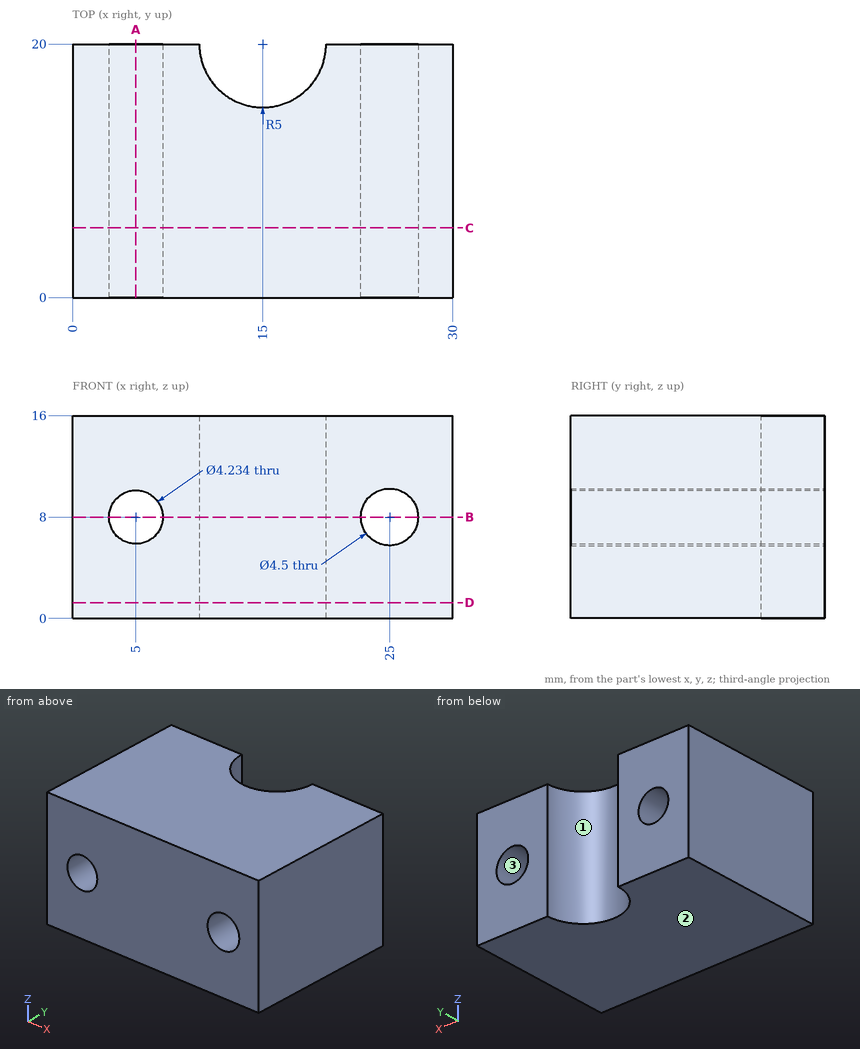
Drawing for the job (mm, zero at the part's lowest x, y, z). Give positions to 0.01 mm unless a question says otherwise; leave off trailing zeros. Order: outer loops, then holes, each group sorted by start corner. A loop starts at its lowest first (then second) coordinate and runs counter-clockwise, first axis right, second up. Notation, with made-up numbers: (88.25, -15) -> (94.25, -15) arc R7 ccw to (94.25, -6) -> close; hole circle Ø11 at (69, -5.75). An arc over 180 degrees is marked (long way). Use one line per item in the form item = value.
(1) Saw through at C-C (y = 5.5). Write the cut outline in (x, z), then the cut area to 3 significant figures.
Solution:
outline = (0, 0) -> (30, 0) -> (30, 16) -> (0, 16) -> close; hole circle Ø4.23 at (5, 8); hole circle Ø4.5 at (25, 8)
area = 450 mm²
(2) Saw through at A-A (x = 5). Write the cut outline in (y, z), then the cut area to 3 significant figures.
Solution:
outline = (0, 0) -> (20, 0) -> (20, 5.88) -> (0, 5.88) -> close; (0, 10.12) -> (20, 10.12) -> (20, 16) -> (0, 16) -> close
area = 235 mm²
(3) Saw through at D-D (z = 1.25). Write the cut outline in (x, y).
Solution:
outline = (0, 0) -> (30, 0) -> (30, 20) -> (20, 20) arc R5 cw to (10, 20) -> (0, 20) -> close
(4) Saw through at B-B (z = 8). Write the cut outline in (x, y), then the cut area to 3 significant figures.
Solution:
outline = (0, 0) -> (2.88, 0) -> (2.88, 20) -> (0, 20) -> close; (7.12, 0) -> (22.75, 0) -> (22.75, 20) -> (20, 20) arc R5 cw to (10, 20) -> (7.12, 20) -> close; (27.25, 0) -> (30, 0) -> (30, 20) -> (27.25, 20) -> close
area = 386 mm²
(5) Pull direction Z, two halves, no side cores. Call the marked faces 1, 2 and 3: +Z half, -Z half, draft (parallel to the pull), parting line (faces both ways), or undercut.
Solution:
face_1 = draft
face_2 = -Z half
face_3 = undercut
(6) Drill centre lines: line 1 (X direction, y = 13, z = 8); line 2 (X direction, y = 16.75, z = 8.5); line 3 (X direction, y = 7, z = 6.25) (1 decimal). Where is each one in solid material? Low to high. Write a range as from..to.
Solution:
line_1 = 0..2.88, 7.12..22.75, 27.25..30
line_2 = 0..2.94, 7.06..11.2, 18.8..22.81, 27.19..30
line_3 = 0..3.8, 6.2..23.6, 26.4..30
